```python
from build123d import *

# Parameters (mm, degrees)
SKETCH1_R                               = 8
BOSS_EXTRUDE1_DEPTH                     = 10
SKETCH2_R                               = 12.5
CUT_EXTRUDE1_DEPTH                      = 10
SKETCH3_R                               = 3.5
CUT_EXTRUDE2_DEPTH                      = 40
SKETCH4_R                               = 6
CUT_EXTRUDE3_DEPTH                      = 6
CIRPATTERN1_COUNT                       = 6
TAP_DRILL_FOR_M10X1_25_TAP1_D           = 8.8
TAP_DRILL_FOR_M10X1_25_TAP1_DEPTH       = 24
TAP_DRILL_FOR_M10X1_25_TAP1_CSINK_D     = 8.85
TAP_DRILL_FOR_M10X1_25_TAP1_CSINK_ANGLE = 90
TAP_DRILL_FOR_M10X1_25_TAP1_TIP         = 2.643786724
CUT_EXTRUDE4_DEPTH                      = 4
FILLET2_R                               = 2
FILLET2_OF_MIRROR5_R                    = 2


with BuildPart() as part:
    # Sketch1 → Boss-Extrude1 (new, symmetric)
    with BuildSketch(Plane.XY):
        with BuildLine():
            Line((-46.348133122, 124.999515212), (-46.348133122, 0))
            Line((-46.348133122, 0), (45.651866878, 0))
            Line((45.651866878, 0), (45.651866878, 124.999515212))
            ThreePointArc((45.651866878, 124.999515212), (-0.348133122, 170.999515212), (-46.348133122, 124.999515212))
        make_face()
        with Locations((-0.348133122, 124.999515212)):
            Circle(SKETCH1_R, mode=Mode.SUBTRACT)
    extrude(amount=BOSS_EXTRUDE1_DEPTH, both=True)

    # Sketch2 → Cut-Extrude1 (cut)
    with BuildSketch(Plane.XY.offset(10)):
        with Locations((-0.348133122, 124.999515212)):
            Circle(SKETCH2_R)
    extrude(amount=-CUT_EXTRUDE1_DEPTH, mode=Mode.SUBTRACT)

    # Sketch3 → Cut-Extrude2 (cut)
    with BuildSketch(Plane.XY.offset(10)):
        with Locations((-0.348133122, 160.999515212)):
            Circle(SKETCH3_R)
    cut_extrude2 = extrude(amount=-CUT_EXTRUDE2_DEPTH, mode=Mode.SUBTRACT)

    # Sketch4 → Cut-Extrude3 (cut)
    with BuildSketch(Plane(origin=(0, 0, -10), x_dir=(-1, 0, 0), z_dir=(0, 0, -1))):
        with Locations((0.348133122, 160.999515212)):
            Circle(SKETCH4_R)
    cut_extrude3 = extrude(amount=-CUT_EXTRUDE3_DEPTH, mode=Mode.SUBTRACT)

    # CirPattern1: Cut-Extrude2, Cut-Extrude3 ×6 about axis
    cirpattern1_axis = Axis((-0.348133122, 124.999515212, 0), (0, 0, 1))
    add([cut_extrude2.rotate(cirpattern1_axis, i * 360 / CIRPATTERN1_COUNT) for i in range(1, CIRPATTERN1_COUNT)], mode=Mode.SUBTRACT)
    add([cut_extrude3.rotate(cirpattern1_axis, i * 360 / CIRPATTERN1_COUNT) for i in range(1, CIRPATTERN1_COUNT)], mode=Mode.SUBTRACT)

    # Tap Drill for M10x1.25 Tap1
    with Locations(Plane(origin=(0, 0, 0), x_dir=(-1, 0, 0), z_dir=(0, -1, 0))):
        with Locations((-29.651866878, 0), (30.348133122, 0)):
            CounterSinkHole(TAP_DRILL_FOR_M10X1_25_TAP1_D / 2, TAP_DRILL_FOR_M10X1_25_TAP1_CSINK_D / 2, depth=TAP_DRILL_FOR_M10X1_25_TAP1_DEPTH, counter_sink_angle=TAP_DRILL_FOR_M10X1_25_TAP1_CSINK_ANGLE)
            with Locations((0, 0, -(TAP_DRILL_FOR_M10X1_25_TAP1_DEPTH + TAP_DRILL_FOR_M10X1_25_TAP1_TIP / 2))):  # 118° drill point
                Cone(0, TAP_DRILL_FOR_M10X1_25_TAP1_D / 2, TAP_DRILL_FOR_M10X1_25_TAP1_TIP, mode=Mode.SUBTRACT)

    # Sketch15 → Cut-Extrude4 (cut)
    with BuildSketch(Plane.XY.offset(10)):
        with BuildLine():
            Line((33.651866878, 12), (33.651866878, 74.205814816))
            ThreePointArc((33.651866878, 74.205814816), (30.703152645, 79.372017984), (24.755315154, 79.460335546))
            ThreePointArc((24.755315154, 79.460335546), (-0.348133122, 72.999515212), (-25.451581398, 79.460335546))
            ThreePointArc((-25.451581398, 79.460335546), (-31.399418888, 79.372017984), (-34.348133122, 74.205814816))
            Line((-34.348133122, 74.205814816), (-34.348133122, 12))
            Line((-34.348133122, 12), (33.651866878, 12))
        make_face()
    cut_extrude4 = extrude(amount=-CUT_EXTRUDE4_DEPTH, mode=Mode.SUBTRACT)

    # Fillet2
    fillet2_edges = [part.edges().sort_by_distance(p)[0] for p in [
        (30.703152645, 79.372017984, 6),
        (33.651866878, 43.102907408, 6),
        (-0.348133122, 12, 6),
        (-34.348133122, 43.102907408, 6),
        (-31.399418888, 79.372017984, 6),
        (-0.348133122, 72.999515212, 6),
    ]]
    fillet(fillet2_edges, radius=FILLET2_R)

    # Mirror5: Cut-Extrude4 across plane
    add(cut_extrude4.mirror(Plane.XY), mode=Mode.SUBTRACT)

    # Fillet2 of Mirror5
    fillet2_of_mirror5_edges = [part.edges().sort_by_distance(p)[0] for p in [
        (30.703152645, 79.372017984, -6),
        (33.651866878, 43.102907408, -6),
        (-0.348133122, 12, -6),
        (-34.348133122, 43.102907408, -6),
        (-31.399418888, 79.372017984, -6),
        (-0.348133122, 72.999515212, -6),
    ]]
    fillet(fillet2_of_mirror5_edges, radius=FILLET2_OF_MIRROR5_R)


solid = part.part
```
Work out the finished part from the listing and answer in its coordinate system (mm). A direction names the side the tool comes from. Round coordinates to 2 decimals unless told otherwise and drop trailing zeros. Loops run counter-clockwise (first coordinate to the right, second up) from the corner with the lowest first, then second, coordinate; pieces in that order, holes last. Notation, with made-up numbers: (9.5, 42.25) -> (41.5, 42.25) arc R19 cw to (41.5, 51.25) -> close; hole circle Ø1 at (10, 67). An arc over 180 degrees is marked (long way). Write each question's results on one line, items separated by ' | '. Start each with the question number.
1. Given pin 1 Ø11 at (x, y) = (-31.53, 143) entering from -Z; pin 2 Ø4 at (x, z) = (-1.5, -6) entering from +Y; pin 3 Ø10 at (x, y) = (-2.5, 37.5) entering from -Z, each flat-ended and moving along its own axis, determine where each tip first touches the part or whether it passes through.
2. Find the intervals of material crossed by probe 1 along Y at (x, z) = (-28.5, -2.75); probe 2 along X at (y, z) = (21, -8.5); probe 3 along Y at (x, z) = (33, -0.75), in increasing order. Write a range as from..to.
3. For a pull along X with two mould halves and no side action, classify faces 5 (the face through (0.43, 166.95, -7.04)), 6 (the face through (0.66, 170.99, 0.14)), 7 (the face through (0.411, 92.416, 3.098)) as +X half, -X half, draft (parallel to the pull), parting line (faces both ways), or undercut.
4. Section A-A (y = 57) is taken. Determine the outline of the cut face in (x, z).
5. Section D-D (x = -39.5) is taken. Determine the outline of the cut face in (y, z), plus the area to 3 significant figures.
6. Section C-C (z = -1.75) is taken. State how many separate pieces and enclosed holes the cut face has, plus the area to 3 significant figures.
7. Section B-B (y = 121.5) is taken. Determine the outline of the cut face in (x, z).
8. A tool of negligible diameter and unlimited length cuts with its end or side. For faces 1 (the face through (30.778, 79.327, -9.014)), 2 (the face through (-0.5, 116.8, 0)), 3 (the face through (-0.8, 164.47, 3.1)), 4 (the face through (25.256, 12.18, -0.193)), from which of +Z, -Z, +X, -X, +Y, -Y can it reach the whole face along a straight path? Write none if from no direction.
Evaluation:
1) pin 1: stops at z = -4 | pin 2: stops at y = 171 | pin 3: stops at z = -6
2) probe 1: y = 24.65..105.24, 108.76..141.24, 144.76..161.38 | probe 2: x = -46.35..-34.35, 33.65..45.65 | probe 3: y = 24.58..104.25, 109.74..140.25, 145.74..156.68
3) face 5: undercut | face 6: parting line | face 7: undercut
4) outline: (-46.35, -10) -> (-34.35, -10) -> (-34.35, -8) arc R2 cw to (-32.35, -6) -> (31.65, -6) arc R2 cw to (33.65, -8) -> (33.65, -10) -> (45.65, -10) -> (45.65, 10) -> (33.65, 10) -> (33.65, 8) arc R2 cw to (31.65, 6) -> (-32.35, 6) arc R2 cw to (-34.35, 8) -> (-34.35, 10) -> (-46.35, 10) -> close
5) outline: (0, -10) -> (149.15, -10) -> (149.15, 10) -> (0, 10) -> close | area: 2,980 mm2
6) separate pieces: 1 | enclosed holes: 7 | area: 14,000 mm2
7) outline: (-46.35, -10) -> (-7.54, -10) -> (-7.54, 0) -> (-12.35, 0) -> (-12.35, 10) -> (-46.35, 10) -> close; (6.85, -10) -> (45.65, -10) -> (45.65, 10) -> (11.65, 10) -> (11.65, 0) -> (6.85, 0) -> close
8) face 1: -Z | face 2: +Z | face 3: +Z, -Z | face 4: -Y
